The listing builds one solid part. Answer for the finished solid, in the listing's coordinates (mm). A direction names the side the tool comes from. Coordinates: 2 decimals unless noted, no trailing zeros. Order: outer loops, then holes, each group sorted by start corner. A loop starts at its lowest first (then second) coordinate and runs counter-clockwise, first axis right, second up. Notation, with made-up numbers: (55, 35.5) -> (108, 35.5) arc R28 cw to (108, 68.5) -> close; hole circle Ø7 at (83.25, 34). An arc over 180 degrees is marked (long way). Answer in a Markdown table with one row per item.
```python
from build123d import *

# Parameters (mm, degrees)
BOSS_EXTRUDE1_DEPTH = 5


with BuildPart() as part:
    # Sketch1 → Boss-Extrude1 (new body)
    with BuildSketch(Plane.YZ):
        Polygon((-30, -28), (-30, 28), (-22, 28), (-22, 33), (-12, 33), (-12, 28), (12, 28), (12, 33), (22, 33), (22, 28), (30, 28), (30, -28), (30, -34), (22, -34), (22, -39), (12, -39), (12, -34), (-12, -34), (-12, -39), (-22, -39), (-22, -34), (-30, -34), align=None)
    extrude(amount=BOSS_EXTRUDE1_DEPTH)


solid = part.part
```
(1) For a pull along Y with two mould halves and no side action, classify faces 4 (the flat face through (2, 12, -37)), 5 (the flat face through (2, -22, 30)), 6 (the flat face through (2, -17, 33)) as released by +Y, released by -Y, zero draft, split by the parting line, or undercut.
Check values:
| item | result |
|---|---|
| face 4 | undercut |
| face 5 | released by -Y |
| face 6 | zero draft |
(2) Find the intervals of material crossed by line 1 along Y through (x, z) = (2.8, 29.5); line 2 along Z through (x, y) = (2.1, 11.5), in increasing order. Write a range as from..to.
Check values:
| item | result |
|---|---|
| line 1 | -22..-12, 12..22 |
| line 2 | -34..28 |
(3) A cutting plane is placed at A-A, the plane x = 1.6. Determine the outline of the cut face in (y, z).
Check values:
| item | result |
|---|---|
| outline | (-30, -34) -> (-22, -34) -> (-22, -39) -> (-12, -39) -> (-12, -34) -> (12, -34) -> (12, -39) -> (22, -39) -> (22, -34) -> (30, -34) -> (30, 28) -> (22, 28) -> (22, 33) -> (12, 33) -> (12, 28) -> (-12, 28) -> (-12, 33) -> (-22, 33) -> (-22, 28) -> (-30, 28) -> close |
(4) Flat-ended cylindrical pins translate along their axes: pin 1 (1.5 mm diameter, centred on x = 1.5, z = -36, fed in from +Y); pin 2 (1.5 mm diameter, centred on x = 2, y = 4.5, fed in from -Z); pin 3 (2.5 mm diameter, centred on x = 1.5, y = -27.5, fed in from +Z). Find the tip coordinate at first contact, or state that the pin passes through.
Check values:
| item | result |
|---|---|
| pin 1 | y = 22 |
| pin 2 | z = -34 |
| pin 3 | z = 28 |
(5) A cutting plane is placed at B-B, the plane y = 3.5. Determine the outline of the cut face in (x, z).
Check values:
| item | result |
|---|---|
| outline | (0, -34) -> (5, -34) -> (5, 28) -> (0, 28) -> close |
(6) Which of the six approach directions +Z, -Z, +X, -X, +Y, -Y give full straight-line access (tool end or side, diameter ignored) to faces 1 (the flat face through (2, 26, 28)), 2 (the flat face through (2, 22, -36)), 3 (the flat face through (2, -26, -34))?
Check values:
| item | result |
|---|---|
| face 1 | +Z, +X, -X, +Y |
| face 2 | -Z, +X, -X, +Y |
| face 3 | -Z, +X, -X, -Y |
